```python
from build123d import *

# Parameters (mm, degrees)
SKETCH_W      = 203.2
SKETCH_H      = 44.45
SKETCH_R      = 2.775
SKETCH_W_2    = 91
SKETCH_H_2    = 28
PAD_DEPTH     = 2.2
SKETCH001_W   = 95
SKETCH001_H   = 32
SKETCH001_W_2 = 91
SKETCH001_H_2 = 28
PAD001_DEPTH  = 87.8
SKETCH002_W   = 95
SKETCH002_H   = 32
SKETCH002_W_2 = 55
SKETCH002_H_2 = 28
PAD002_DEPTH  = 2


with BuildPart() as part:
    # Sketch → Pad (new body)
    with BuildSketch(Plane.XY):
        Rectangle(SKETCH_W, SKETCH_H)
        with Locations((-93.6625, 15.875)):
            Circle(SKETCH_R, mode=Mode.SUBTRACT)
        with Locations((-93.6625, -15.875)):
            Circle(SKETCH_R, mode=Mode.SUBTRACT)
        with Locations((93.6625, 15.875)):
            Circle(SKETCH_R, mode=Mode.SUBTRACT)
        with Locations((93.6625, -15.875)):
            Circle(SKETCH_R, mode=Mode.SUBTRACT)
        Rectangle(SKETCH_W_2, SKETCH_H_2, mode=Mode.SUBTRACT)
    extrude(amount=PAD_DEPTH)

    # Sketch001 (on Face14 of Pad) → Pad001 (join)
    with BuildSketch(Plane.XY.offset(2.2)):
        Rectangle(SKETCH001_W, SKETCH001_H)
        Rectangle(SKETCH001_W_2, SKETCH001_H_2, mode=Mode.SUBTRACT)
    extrude(amount=PAD001_DEPTH)

    # Sketch002 (on Face23 of Pad001) → Pad002 (join)
    with BuildSketch(Plane.XY.offset(90)):
        Rectangle(SKETCH002_W, SKETCH002_H)
        Rectangle(SKETCH002_W_2, SKETCH002_H_2, mode=Mode.SUBTRACT)
    extrude(amount=PAD002_DEPTH)


solid = part.part
```
Work out the finished part from the listing and answer in its coordinate system (mm). A direction names the side the tool comes from. Give positions to 0.01 mm unless a question says otherwise; leave off trailing zeros. Write each loop counter-clockwise with the first axis right and the second up, starting at its lowest first coordinate (ties: lowest second). Pieces come first, ordered by that corner, then holes. Notation, with made-up numbers: (40, 21) - (54, 21) arc R25 cw to (54, 52) - close; hole circle Ø3 at (50, -25.5). An arc over 180 degrees is marked (long way). Use one line per item in the form item = value.
1. A cutting plane is placed at C-C (z = 22.5). Write down the section's boundary in (x, y), and give its area (3 significant figures).
Filled in:
outline = (-47.5, -16) - (47.5, -16) - (47.5, 16) - (-47.5, 16) - close; hole (-45.5, -14) - (45.5, -14) - (45.5, 14) - (-45.5, 14) - close
area = 492 mm^2
2. Consider L1, parallel to X at y = -4.5, z = 16; L2, parallel to Y at x = 7.5, z = 39; L3, parallel to X at y = -15, z = 28. Determine where each line is inside the solid, lowest interval first.
Filled in:
L1 = -47.5 to -45.5, 45.5 to 47.5
L2 = -16 to -14, 14 to 16
L3 = -47.5 to 47.5
3. Each of these flat-tipped pins is pushed along its axis until it touches: pin 1 Ø1 at (x, z) = (-28.5, 36) entering from +Y; pin 2 Ø0.6 at (y, z) = (-2, 91) entering from -X; pin 3 Ø9 at (x, y) = (-93.66, 15.88) entering from +Z. Where does it stop, or does it pass through?
Filled in:
pin_1 = 16
pin_2 = -47.5
pin_3 = 2.2
4. A cutting plane is placed at A-A (x = 7). Write down the section's boundary in (y, z) (3 decimals), and give its area (3 significant figures).
Filled in:
outline = (-22.225, 0) - (-14, 0) - (-14, 92) - (-16, 92) - (-16, 2.2) - (-22.225, 2.2) - close; (14, 0) - (22.225, 0) - (22.225, 2.2) - (16, 2.2) - (16, 92) - (14, 92) - close
area = 395 mm^2
5. Determine the mould class of faces 1 (the face through (47.5, 0, 46)), 2 (the face through (-1, -14, 45)), 3 (the face through (-1, -16, 46)) for opening direction Y: released by +Y, released by -Y, zero draft, split by the parting line, or undercut.
Filled in:
face_1 = zero draft
face_2 = undercut
face_3 = released by -Y
6. A cutting plane is placed at D-D (x = -41). Write down the section's boundary in (y, z) (3 decimals), and give its area (3 significant figures).
Filled in:
outline = (-22.225, 0) - (-14, 0) - (-14, 90) - (14, 90) - (14, 0) - (22.225, 0) - (22.225, 2.2) - (16, 2.2) - (16, 92) - (-16, 92) - (-16, 2.2) - (-22.225, 2.2) - close
area = 451 mm^2
7. A cutting plane is placed at B-B (y = 5.5). Write down the section's boundary in (x, z).
Filled in:
outline = (-101.6, 0) - (-45.5, 0) - (-45.5, 90) - (-27.5, 90) - (-27.5, 92) - (-47.5, 92) - (-47.5, 2.2) - (-101.6, 2.2) - close; (27.5, 90) - (45.5, 90) - (45.5, 0) - (101.6, 0) - (101.6, 2.2) - (47.5, 2.2) - (47.5, 92) - (27.5, 92) - close
8. For faces 4 (the face through (-37, 0, 90)), 5 (the face through (-47.5, 0, 46)), 6 (the face through (-1, 16, 46)), determine the directions among +Z, -Z, +X, -X, +Y, -Y from which every point of the face is accessible in a straight line to the end or side of a thin tool.
Filled in:
face_4 = -Z
face_5 = +Z, -X, +Y, -Y
face_6 = +Z, +X, -X, +Y
